```python
from build123d import *

# Parameters (mm, degrees)
SKETCH1_W                                      = 28
SKETCH1_H                                      = 30
BOSS_EXTRUDE1_DEPTH                            = 11
CBORE_FOR_8_SOCKET_HEAD_CAP_SCREW3_D           = 4.4958
CBORE_FOR_8_SOCKET_HEAD_CAP_SCREW3_DEPTH       = 11
CBORE_FOR_8_SOCKET_HEAD_CAP_SCREW3_CBORE_D     = 7.9375
CBORE_FOR_8_SOCKET_HEAD_CAP_SCREW3_CBORE_DEPTH = 4.1656
F_8_32_TAPPED_HOLE1_AT_2_COUNT                 = 2
F_8_32_TAPPED_HOLE1_AT_2_PITCH                 = 20
F_1_8_0_1250_DOWEL_HOLE1_AT_2_COUNT            = 2
F_1_8_0_1250_DOWEL_HOLE1_AT_2_PITCH            = 10


with BuildPart() as part:
    # Sketch1 → Boss-Extrude1 (new body)
    with BuildSketch(Plane.XY):
        with Locations((14, 0)):
            Rectangle(SKETCH1_W, SKETCH1_H)
    extrude(amount=BOSS_EXTRUDE1_DEPTH)

    # Sketch16 → CBORE for M5 Hex Head Bolt1 (revolve, cut)
    with BuildSketch(Plane.YZ.offset(14)):
        Polygon((0, 0), (0, 11), (4, 11), (4, 3.25), (4.25, 3), (5.5, 3), (5.5, 1), (6.5, 0), align=None)
    revolve(axis=Axis((14, 0, -6.35), (0, 0, 1)), mode=Mode.SUBTRACT)

    # CBORE for #8 Socket Head Cap Screw3
    with Locations(Plane.XY.offset(11)):
        with Locations((23.5, 0), (4.5, 0), (14, 9.5), (14, -9.5)):
            CounterBoreHole(CBORE_FOR_8_SOCKET_HEAD_CAP_SCREW3_D / 2, CBORE_FOR_8_SOCKET_HEAD_CAP_SCREW3_CBORE_D / 2, CBORE_FOR_8_SOCKET_HEAD_CAP_SCREW3_CBORE_DEPTH, depth=CBORE_FOR_8_SOCKET_HEAD_CAP_SCREW3_DEPTH)

    # Sketch13 → #8-32 Tapped Hole1 (revolve, cut)
    with BuildSketch(Plane(origin=(4, 15, 5.5), x_dir=(0, 0, 1), z_dir=(1, 0, 0))):
        Polygon((0, 0), (0, 11.037806461), (1.7272, 10), (1.7272, 0), align=None)
    f_8_32_tapped_hole1 = revolve(axis=Axis((4, 21.35, 5.5), (0, -1, 0)), mode=Mode.SUBTRACT)

    # #8-32 Tapped Hole1 at 2: #8-32 Tapped Hole1 ×2
    with Locations(*[(i * F_8_32_TAPPED_HOLE1_AT_2_PITCH, 0, 0) for i in range(1, F_8_32_TAPPED_HOLE1_AT_2_COUNT)]):
        add(f_8_32_tapped_hole1, mode=Mode.SUBTRACT)

    # Sketch20 → 1/8 (0.1250) Dowel Hole1 (revolve, cut)
    with BuildSketch(Plane(origin=(9, 15, 4), x_dir=(0, 0, 1), z_dir=(1, 0, 0))):
        Polygon((0, 0), (0, 5.953866233), (1.5875, 5), (1.5875, 0), align=None)
    f_1_8_0_1250_dowel_hole1 = revolve(axis=Axis((9, 21.35, 4), (0, -1, 0)), mode=Mode.SUBTRACT)

    # 1/8 (0.1250) Dowel Hole1 at 2: 1/8 (0.1250) Dowel Hole1 ×2
    with Locations(*[(i * F_1_8_0_1250_DOWEL_HOLE1_AT_2_PITCH, 0, 0) for i in range(1, F_1_8_0_1250_DOWEL_HOLE1_AT_2_COUNT)]):
        add(f_1_8_0_1250_dowel_hole1, mode=Mode.SUBTRACT)

    # Mirror1: 1/8 (0.1250) Dowel Hole1, #8-32 Tapped Hole1 across plane
    add(f_1_8_0_1250_dowel_hole1.mirror(Plane.ZX), mode=Mode.SUBTRACT)
    add(f_8_32_tapped_hole1.mirror(Plane.ZX), mode=Mode.SUBTRACT)

    # Mirror1 copy 1 sketch → Mirror1 copy 1 (revolve, cut)
    with BuildSketch(Plane(origin=(19, -15, 4), x_dir=(0, 0, 1), z_dir=(1, 0, 0))):
        Polygon((0, 0), (0, -5.953866233), (1.5875, -5), (1.5875, 0), align=None)
    revolve(axis=Axis((19, -21.35, 4), (0, -1, 0)), mode=Mode.SUBTRACT)

    # Mirror1 copy 2 sketch → Mirror1 copy 2 (revolve, cut)
    with BuildSketch(Plane(origin=(24, -15, 5.5), x_dir=(0, 0, 1), z_dir=(1, 0, 0))):
        Polygon((0, 0), (0, -11.037806461), (1.7272, -10), (1.7272, 0), align=None)
    revolve(axis=Axis((24, -21.35, 5.5), (0, -1, 0)), mode=Mode.SUBTRACT)


solid = part.part
```
Geometry check sheet. Reference: the model listing, model coordinates, mm. A direction names the side the tool comes from. Give positions to 0.01 mm unless a question says otherwise; leave off trailing zeros. Loops run counter-clockwise (first coordinate to the right, second up) from the corner with the lowest first, then second, coordinate; pieces in that order, holes last. Notation, with made-up numbers: M 10.5,8.25 L 38.5,8.25 A21 ccw 38.5,33.25 Z; hole C 85,-10 d5. An arc over 180 degrees is marked long. Write item = value, one per line.
(1) Release check for a two-part mould opening along X. For faces 5 (the face through (28, 0, 5)), 6 (the face through (16, 8, 6.834)), 7 (the face through (14, 15, 5)) record: released by +X, released by -X, zero draft, split by the parting line, or undercut.
Answer below:
face_5 = released by +X
face_6 = undercut
face_7 = zero draft
(2) Sectioned sample at C-C, the plane z = 9.25. Record the cut outline in (x, y), plus the area to 3 significant figures.
Answer below:
outline = M 0,-15 L 28,-15 L 28,15 L 0,15 Z; hole C 4.5,0 d7.94; hole C 14,0 d8; hole C 14,-9.5 d7.94; hole C 14,9.5 d7.94; hole C 23.5,0 d7.94
area = 592 mm2
(3) Sectioned sample at A-A, the plane y = 8.5. Record the cut outline in (x, z).
Answer below:
outline = M 0,0 L 11.99,0 L 11.99,6.83 L 10.16,6.83 L 10.16,11 L 0,11 Z; M 16.01,0 L 28,0 L 28,11 L 17.84,11 L 17.84,6.83 L 16.01,6.83 Z; hole C 4,5.5 d3.45; hole C 24,5.5 d3.45
(4) Gauge pin test, flat ends, axial feed: pin 1 Ø3 at (x, z) = (24, 4.5) entering from +Y; pin 2 Ø6.5 at (x, y) = (23.5, 0) entering from +Z; pin 3 Ø6.5 at (x, y) = (14, 0) entering from +Z; pin 4 Ø1.9 at (x, z) = (19, 4) entering from +Y. Record the tip position at first contact, or that the pin passes through.
Answer below:
pin_1 = 15
pin_2 = 6.83
pin_3 = through
pin_4 = 9.62
(5) Material ranges on line 1 (Y direction, x = 14, z = 2.75); line 2 (Y direction, x = 14, z = 4.5); line 3 (Z direction, x = 9, y = 12.25), recorded low to high. Write a range as [from, to].
Answer below:
line_1 = [-15, -11.75], [-7.25, -5.5], [5.5, 7.25], [11.75, 15]
line_2 = [-15, -11.75], [-7.25, -4], [4, 7.25], [11.75, 15]
line_3 = [0, 2.41], [5.59, 11]
(6) Tool access check on faces 1 (the face through (8.523, -12.535, 5.514)), 2 (the face through (27.166, -1.52, 8.946)), 3 (the face through (20.55, 12.54, 3.66)), 4 (the face through (18, -2, 3)). Record the directions out of +Z, -Z, +X, -X, +Y, -Y that give a thin tool (end or side, any length) a straight path to the whole face; none if there is none.
Answer below:
face_1 = -Y
face_2 = +Z
face_3 = +Y
face_4 = -Z
(7) Sectioned sample at B-B, the plane x = 14. State how many separate pieces and enclosed holes the cut face has, plus the area to 3 significant figures.
Answer below:
separate_pieces = 4
enclosed_holes = 0
area = 104 mm2
